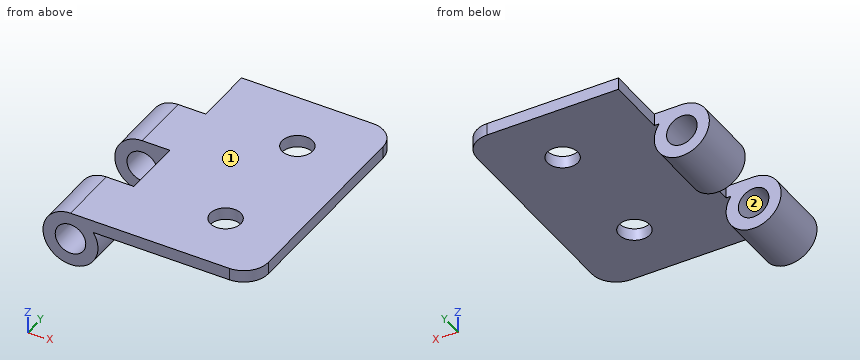
from build123d import *

# Parameters (mm, degrees)
SKETCH_1_R          = 2.5
EXTRUDE_1_DEPTH     = 40
CUT_EXTRUDE_1_REACH = 52.804
SKETCH_2_R          = 2.5
SKETCH_3_W          = 9
SKETCH_3_H          = 10
CUT_EXTRUDE_2_DEPTH = 20
FILLET_1_R          = 4


with BuildPart() as part:
    # 草图1 → 凸台-拉伸1 (new body)
    with BuildSketch(Plane(origin=(0, 0, 0), x_dir=(1, 0, 0), z_dir=(0, 1, 0))):
        with BuildLine():
            Line((0, -4.5), (30, -4.5))
            Line((30, -4.5), (30, -2.5))
            Line((30, -2.5), (3.741657387, -2.5))
            ThreePointArc((3.741657387, -2.5), (-2.121320344, 3.968626967), (0, -4.5))
        make_face()
        with Locations(Location((0, 0, 0), (0, 0, 270))):
            Circle(SKETCH_1_R, mode=Mode.SUBTRACT)
    extrude(amount=EXTRUDE_1_DEPTH)

    # 草图2 → 切除-拉伸1 (cut, up to next)
    with BuildSketch(Plane.XY.offset(4.5), mode=Mode.PRIVATE) as cut_extrude_1_sk1:
        with Locations((19.5, 30)):
            Circle(SKETCH_2_R)
    cut_extrude_1_tool1 = extrude(cut_extrude_1_sk1.sketch, amount=-CUT_EXTRUDE_1_REACH, mode=Mode.PRIVATE) & part.part
    # 草图2 → 切除-拉伸1 (cut, up to next)
    with BuildSketch(Plane.XY.offset(4.5), mode=Mode.PRIVATE) as cut_extrude_1_sk2:
        with Locations((19.5, 10)):
            Circle(SKETCH_2_R)
    cut_extrude_1_tool2 = extrude(cut_extrude_1_sk2.sketch, amount=-CUT_EXTRUDE_1_REACH, mode=Mode.PRIVATE) & part.part
    add(cut_extrude_1_tool1.solids().sort_by_distance((19.5, 30, 4.5))[0], mode=Mode.SUBTRACT)
    add(cut_extrude_1_tool2.solids().sort_by_distance((19.5, 10, 4.5))[0], mode=Mode.SUBTRACT)

    # 草图3 → 切除-拉伸2 (cut, symmetric)
    with BuildSketch(Plane(origin=(0, 0, 2.5), x_dir=(-1, 0, 0), z_dir=(0, 0, -1))):
        with Locations((0, 35)):
            Rectangle(SKETCH_3_W, SKETCH_3_H)
        with Locations((0, 15)):
            Rectangle(SKETCH_3_W, SKETCH_3_H)
    extrude(amount=CUT_EXTRUDE_2_DEPTH, both=True, mode=Mode.SUBTRACT)

    # 圆角1
    fillet_1_edges = [part.edges().sort_by_distance(p)[0] for p in [
        (30, 40, 3.5),
        (30, 0, 3.5),
    ]]
    fillet(fillet_1_edges, radius=FILLET_1_R)


solid = part.part
Here's how the part is built. I have some questions about the finished solid (model axes, mm). Face numbers are marked on the shaded views. Round coordinates to 2 decimals unless told otherwise and drop trailing zeros. Loops run counter-clockwise (first coordinate to the right, second up) from the corner with the lowest first, then second, coordinate; pieces in that order, holes last. Notation, with made-up numbers: (77, -36) - (107, -36) arc R20 cw to (107, -21) - close; hole circle Ø5 at (-16.5, 15). An arc over 180 degrees is marked (long way). One line per question, with ' | ' between items. Start each with the question number.
Q1. Will these pins go through, and if not, where does the flat tip stop? pin 1 (0.6 mm diameter, centred on y = 36, z = 3, fed in from -X); pin 2 (12 mm diameter, centred on x = 20, y = 6.5, fed in from -Z); pin 3 (1.5 mm diameter, centred on y = 8.5, z = -2, fed in from +X).
Q2. I want a section at C-C (z = 3.75). Write out the boundary of the cut face in (x, y), then the cut area to 3 significant figures.
Q3. I want a section at A-A (z = 0). Write out the boundary of the cut face in (x, y), then the cut area to 3 significant figures.
Q4. Please list where these lines run through material, in increasing order: line 1 (Y direction, x = 19.5, z = 3.85); line 2 (Y direction, x = 1, z = -3.5); line 3 (X direction, y = 4.25, z = 0). Write a range as [from, to].
Q5. I want a section at B-B (x = 19.5). Write out the boundary of the cut face in (y, z).
Q6. We'd pull the mould along Z, two halves only. Please class the marked faces 1 and 2: +Z half, -Z half, draft (parallel to the pull), parting line (faces both ways), or undercut.
Q7. I want a section at D-D (y = 35). Write out the boundary of the cut face in (x, z), then the cut area to 3 significant figures.
Response values:
1) pin 1: stops at x = 4.5 | pin 2: stops at z = 2.5 | pin 3: stops at x = 4.32
2) outline: (-2.49, 0) - (26, 0) arc R4 ccw to (30, 4) - (30, 36) arc R4 ccw to (26, 40) - (4.5, 40) - (4.5, 30) - (-2.49, 30) - (-2.49, 20) - (4.5, 20) - (4.5, 10) - (-2.49, 10) - close; hole circle Ø5 at (19.5, 10); hole circle Ø5 at (19.5, 30) | area: 1,110 mm²
3) outline: (-4.5, 0) - (-2.5, 0) - (-2.5, 10) - (-4.5, 10) - close; (-4.5, 20) - (-2.5, 20) - (-2.5, 30) - (-4.5, 30) - close; (2.5, 0) - (4.5, 0) - (4.5, 10) - (2.5, 10) - close; (2.5, 20) - (4.5, 20) - (4.5, 30) - (2.5, 30) - close | area: 80.0 mm²
4) line 1: y = [0, 7.5], [12.5, 27.5], [32.5, 40] | line 2: y = [0, 10], [20, 30] | line 3: x = [-4.5, -2.5], [2.5, 4.5]
5) outline: (0, 2.5) - (7.5, 2.5) - (7.5, 4.5) - (0, 4.5) - close; (12.5, 2.5) - (27.5, 2.5) - (27.5, 4.5) - (12.5, 4.5) - close; (32.5, 2.5) - (40, 2.5) - (40, 4.5) - (32.5, 4.5) - close
6) face 1: +Z half | face 2: undercut
7) outline: (4.5, 2.5) - (30, 2.5) - (30, 4.5) - (4.5, 4.5) - close | area: 51.0 mm²
